```python
from build123d import *

# Parameters (mm, degrees)
F0_R     = 7.865612
F1_DEPTH = 12.7
F2_R     = 6.403691
F3_DEPTH = 44.45
F4_SIZE  = 6.35
F5_SIZE  = 6.35


with BuildPart() as f1:
    # F0 (on Top) → F1 (new body, symmetric)
    with BuildSketch(Plane.XY):
        with BuildLine():
            Line((-82.702047, -12.7), (-19.202047, -12.7))
            ThreePointArc((-19.202047, -12.7), (-10.221791, -16.419744), (-6.502047, -25.4))
            ThreePointArc((-6.502047, -25.4), (-2.782303, -34.380256), (6.197953, -38.1))
            Line((6.197953, -38.1), (95.097953, -38.1))
            Line((95.097953, -38.1), (95.097953, -12.7))
            Line((95.097953, -12.7), (31.597953, -12.7))
            ThreePointArc((31.597953, -12.7), (22.617697, -8.980256), (18.897953, 0))
            ThreePointArc((18.897953, 0), (22.617697, 8.980256), (31.597953, 12.7))
            Line((31.597953, 12.7), (95.097953, 12.7))
            Line((95.097953, 12.7), (95.097953, 38.1))
            Line((95.097953, 38.1), (6.197953, 38.1))
            ThreePointArc((6.197953, 38.1), (-2.782303, 34.380256), (-6.502047, 25.4))
            ThreePointArc((-6.502047, 25.4), (-10.221791, 16.419744), (-19.202047, 12.7))
            Line((-19.202047, 12.7), (-82.702047, 12.7))
            Line((-82.702047, 12.7), (-82.702047, -12.7))
        make_face()
        with Locations((-70.002047, 0)):
            Circle(F0_R, mode=Mode.SUBTRACT)
    extrude(amount=F1_DEPTH, both=True)

    # F2 (on Front) → F3 (cut, symmetric)
    with BuildSketch(Plane.XZ):
        with Locations((82.397953, 0)):
            Circle(F2_R)
    extrude(amount=F3_DEPTH, both=True, mode=Mode.SUBTRACT)

    # F4
    f4_edges = [f1.edges().sort_by_distance(p)[0] for p in [
        (95.097953, -25.4, 12.7),
        (95.097953, -25.4, -12.7),
    ]]
    chamfer(f4_edges, length=F4_SIZE)

    # F5
    f5_edges = [f1.edges().sort_by_distance(p)[0] for p in [
        (95.097953, 25.4, 12.7),
        (95.097953, 25.4, -12.7),
    ]]
    chamfer(f5_edges, length=F5_SIZE)


solid = f1.part
```
Part model, mm, in its own coordinate system. A direction names the side the tool comes from. Round coordinates to 2 decimals unless told otherwise and drop trailing zeros. Loops run counter-clockwise (first coordinate to the right, second up) from the corner with the lowest first, then second, coordinate; pieces in that order, holes last. Notation, with made-up numbers: (80, 11) -> (91, 11) arc R9 ccw to (91, 16) -> close; hole circle Ø8 at (32, -2). An arc over 180 degrees is marked (long way). Use CSV: the item, a comma, the result in double quotes. Start each with the question number.
1) Drop flat-ended pins along their axis: P1, Ø12, axis at y = -22.5, z = 5, coming from the -X side; P2, Ø10, axis at x = -21, z = -6.5, coming from the -Y side; P3, Ø12.5, axis at x = -66, z = 5, coming from the +Y side; P4, Ø6, axis at y = 18.5, z = -8, coming from the +X side. Give the stop position or say it passes through.
2) Cut at D-D, the plane y = 27. Write the cut outline in (x, z), plus the area to 3 significant figures.
3) Cut at B-B, the plane x = 22.5. Write the cut outline in (y, z).
4) Cut at C-C, the plane y = 6. Write the cut outline in (x, z).
5) Which spindle directions (+Z, -Z, +X, -X, +Y, -Y) get a long thin tool onto all of the face, cutting with end or side? Do faces 4 (the flat face through (91.97, -25.58, -9.48)), 5 (the flat face through (-51, 12.7, 0)), 6 (the flat face through (-51, -12.7, 0)), 7 (the flat face through (64, -12.7, 0)). Say none if no direction does.
6) Cut at A-A, the plane z = 0. Write the cut outline in (x, y).
7) Pull direction X, two halves, no side cores. Call faces 1 (the flat face through (21, 9, 12.7)), 2 (the cylindrical face through (-76.24, -4.79, -0.18)), 3 (the flat face through (95.098, 25, 0)): +X half, -X half, draft (parallel to the pull), parting line (faces both ways), or undercut.
8) Wall check: L1, parallel to Y at x = 77, z = -11; L2, parallel to X at y = -1, z = -7.5; L3, parallel to Y at x = -28, z = 2.5. Give the ranges that are in metal, low to high. Write a range as [from, to].
Determined:
1,P1,"stops at x = -10.14"
1,P2,"stops at y = -13.11"
1,P3,"stops at y = 12.7"
1,P4,"stops at x = 95.1"
2,outline,"(-6.4, -12.7) -> (88.75, -12.7) -> (95.1, -6.35) -> (95.1, 6.35) -> (88.75, 12.7) -> (-6.4, 12.7) -> close; hole circle Ø12.81 at (82.4, 0)"
2,area,"2,410 mm2"
3,outline,"(-38.1, -12.7) -> (-8.86, -12.7) -> (-8.86, 12.7) -> (-38.1, 12.7) -> close; (8.86, -12.7) -> (38.1, -12.7) -> (38.1, 12.7) -> (8.86, 12.7) -> close"
4,outline,"(-82.7, -12.7) -> (-75.09, -12.7) -> (-75.09, 12.7) -> (-82.7, 12.7) -> close; (-64.92, -12.7) -> (20.4, -12.7) -> (20.4, 12.7) -> (-64.92, 12.7) -> close"
5,face 4,"-Z, +X, +Y, -Y"
5,face 5,"+Z, -Z, -X, +Y"
5,face 6,"+Z, -Z, -X, -Y"
5,face 7,"+Z, -Z, +X"
6,outline,"(-82.7, -12.7) -> (-19.2, -12.7) arc R12.7 cw to (-6.5, -25.4) arc R12.7 ccw to (6.2, -38.1) -> (75.99, -38.1) -> (75.99, -12.7) -> (31.6, -12.7) arc R12.7 cw to (31.6, 12.7) -> (75.99, 12.7) -> (75.99, 38.1) -> (6.2, 38.1) arc R12.7 ccw to (-6.5, 25.4) arc R12.7 cw to (-19.2, 12.7) -> (-82.7, 12.7) -> close; (88.8, -38.1) -> (95.1, -38.1) -> (95.1, -12.7) -> (88.8, -12.7) -> close; (88.8, 12.7) -> (95.1, 12.7) -> (95.1, 38.1) -> (88.8, 38.1) -> close; hole circle Ø15.73 at (-70, 0)"
7,face 1,"draft"
7,face 2,"undercut"
7,face 3,"+X half"
8,L1,"y = [-38.1, -12.7], [12.7, 38.1]"
8,L2,"x = [-82.7, -77.8], [-62.2, 18.94]"
8,L3,"y = [-12.7, 12.7]"
